The listing builds one solid part. Answer for the finished solid, in the listing's coordinates (mm). Face numbers are marked on the shaded views. Round coordinates to 2 decimals unless told otherwise and drop trailing zeros. Order: outer loops, then holes, each group sorted by start corner. A loop starts at its lowest first (then second) coordinate and runs counter-clockwise, first axis right, second up. Notation, with made-up numbers: (75, 87) -> (125, 87) arc R21 cw to (125, 103) -> close; hole circle Ø11 at (-21, 86). An arc over 180 degrees is marked (long way). Answer in a Markdown table with one row per item. Add a question column.
```python
from build123d import *
from build123d.topology import SkipClean

# Parameters (mm, degrees)
SKETCH1_R           = 76.2
BOSS_EXTRUDE1_DEPTH = 6.35
CUT_EXTRUDE2_START  = -6.35
SKETCH2_R           = 4.7625
SKETCH2_R_2         = 19.05
CUT_EXTRUDE2_DEPTH  = 6.35
BOSS_EXTRUDE2_DEPTH = 3
SKETCH4_R           = 1.5
SKETCH4_R_2         = 1.25
CUT_EXTRUDE3_DEPTH  = 86.348763
FILLET1_R           = 2.54
SKETCH5_R           = 2.5
CUT_EXTRUDE4_DEPTH  = 2.85


with BuildPart() as part:
    # Sketch1 → Boss-Extrude1 (new body)
    with BuildSketch(Plane(origin=(0, 0, 0), x_dir=(1, 0, 0), z_dir=(0, 1, 0))):
        with Locations(Location((0, 0, 0), (0, 0, 270))):
            Circle(SKETCH1_R)
    extrude(amount=BOSS_EXTRUDE1_DEPTH)

    # Sketch2 → Cut-Extrude2 (cut)
    with BuildSketch(Plane(origin=(0, 6.35, 0), x_dir=(1, 0, 0), z_dir=(0, 1, 0)).offset(CUT_EXTRUDE2_START)):
        with BuildLine():
            ThreePointArc((61.150771, -23.195291), (0, -37.290064), (-61.150771, -23.195291))
            ThreePointArc((-61.150771, -23.195291), (-72.108092, -13.824804), (-76.2, 0))
            ThreePointArc((-76.2, 0), (0, -76.2), (76.2, 0))
            ThreePointArc((76.2, 0), (72.108092, -13.824804), (61.150771, -23.195291))
        make_face()
        with BuildLine():
            ThreePointArc((-61.150771, 23.195291), (0, 37.290064), (61.150771, 23.195291))
            ThreePointArc((61.150771, 23.195291), (72.108092, 13.824804), (76.2, 0))
            ThreePointArc((76.2, 0), (0, 76.2), (-76.2, 0))
            ThreePointArc((-76.2, 0), (-72.108092, 13.824804), (-61.150771, 23.195291))
        make_face()
        with Locations(Location((-50.8, 0, 0), (0, 0, 270))):
            Circle(SKETCH2_R)
        with Locations(Location((50.8, 0, 0), (0, 0, 270))):
            Circle(SKETCH2_R)
        with Locations(Location((0, 0, 0), (0, 0, 270))):
            Circle(SKETCH2_R_2)
    extrude(amount=CUT_EXTRUDE2_DEPTH, mode=Mode.SUBTRACT)

    # Sketch3 → Boss-Extrude2 (add)
    with SkipClean():  # the faces are left unmerged after this step: merging them gives an invalid solid
        with BuildSketch(Plane(origin=(0, 6.35, 0), x_dir=(1, 0, 0), z_dir=(0, 1, 0))):
            with BuildLine():
                Line((-38.5, 4.75), (-38.5, -4.75))
                Line((-38.5, -4.75), (-38.5, -11.25))
                Line((-38.5, -11.25), (-38.5, -16))
                Line((-38.5, -16), (-18, -16))
                Line((-18, -16), (-11.5, -16))
                Line((-11.5, -16), (-10.339367, -16))
                ThreePointArc((-10.339367, -16), (-13.611535, -13.327739), (-16.214268, -10))
                Line((-16.214268, -10), (-31.096327, -10))
                Line((-31.096327, -10), (-32.5, -10))
                Line((-32.5, -10), (-32.5, -8.522949))
                Line((-32.5, -8.522949), (-32.5, 8.425596))
                Line((-32.5, 8.425596), (-32.5, 10))
                Line((-32.5, 10), (-31.027855, 10))
                Line((-31.027855, 10), (-16.214268, 10))
                ThreePointArc((-16.214268, 10), (-13.611535, 13.327739), (-10.339367, 16))
                Line((-10.339367, 16), (-11.5, 16))
                Line((-11.5, 16), (-18, 16))
                Line((-18, 16), (-38.5, 16))
                Line((-38.5, 16), (-38.5, 11.25))
                Line((-38.5, 11.25), (-38.5, 4.75))
            make_face()
        extrude(amount=BOSS_EXTRUDE2_DEPTH)

    # Sketch4 → Cut-Extrude3 (cut, through all)
    # profile 1 of 12: a face of its own
    with SkipClean():  # the faces are left unmerged after this step: merging them gives an invalid solid
        with BuildSketch(Plane(origin=(0, 9.35, 0), x_dir=(1, 0, 0), z_dir=(0, 1, 0))):
            with Locations(Location((-30.75, -13.5, 0), (0, 0, 270))):
                Circle(SKETCH4_R)
            with Locations((-30.75, -13.5)):
                Circle(SKETCH4_R_2, mode=Mode.SUBTRACT)
        # profile 2 of 12: a face of its own
        with BuildSketch(Plane(origin=(0, 9.35, 0), x_dir=(1, 0, 0), z_dir=(0, 1, 0))):
            with Locations((-30.75, -13.5)):
                Circle(SKETCH4_R_2)
        # profile 3 of 12: a face of its own
        with BuildSketch(Plane(origin=(0, 9.35, 0), x_dir=(1, 0, 0), z_dir=(0, 1, 0))):
            with Locations(Location((-22.75, -13.5, 0), (0, 0, 270))):
                Circle(SKETCH4_R)
            with Locations((-22.75, -13.5)):
                Circle(SKETCH4_R_2, mode=Mode.SUBTRACT)
        # profile 4 of 12: a face of its own
        with BuildSketch(Plane(origin=(0, 9.35, 0), x_dir=(1, 0, 0), z_dir=(0, 1, 0))):
            with Locations((-22.75, -13.5)):
                Circle(SKETCH4_R_2)
        # profile 5 of 12: a face of its own
        with BuildSketch(Plane(origin=(0, 9.35, 0), x_dir=(1, 0, 0), z_dir=(0, 1, 0))):
            with Locations(Location((-36, -8, 0), (0, 0, 270))):
                Circle(SKETCH4_R)
            with Locations((-36, -8)):
                Circle(SKETCH4_R_2, mode=Mode.SUBTRACT)
        # profile 6 of 12: a face of its own
        with BuildSketch(Plane(origin=(0, 9.35, 0), x_dir=(1, 0, 0), z_dir=(0, 1, 0))):
            with Locations((-36, -8)):
                Circle(SKETCH4_R_2)
        # profile 7 of 12: a face of its own
        with BuildSketch(Plane(origin=(0, 9.35, 0), x_dir=(1, 0, 0), z_dir=(0, 1, 0))):
            with Locations(Location((-36, 8, 0), (0, 0, 270))):
                Circle(SKETCH4_R)
            with Locations((-36, 8)):
                Circle(SKETCH4_R_2, mode=Mode.SUBTRACT)
        # profile 8 of 12: a face of its own
        with BuildSketch(Plane(origin=(0, 9.35, 0), x_dir=(1, 0, 0), z_dir=(0, 1, 0))):
            with Locations((-36, 8)):
                Circle(SKETCH4_R_2)
        # profile 9 of 12: a face of its own
        with BuildSketch(Plane(origin=(0, 9.35, 0), x_dir=(1, 0, 0), z_dir=(0, 1, 0))):
            with Locations(Location((-30.75, 13.5, 0), (0, 0, 270))):
                Circle(SKETCH4_R)
            with Locations((-30.75, 13.5)):
                Circle(SKETCH4_R_2, mode=Mode.SUBTRACT)
        # profile 10 of 12: a face of its own
        with BuildSketch(Plane(origin=(0, 9.35, 0), x_dir=(1, 0, 0), z_dir=(0, 1, 0))):
            with Locations((-30.75, 13.5)):
                Circle(SKETCH4_R_2)
        # profile 11 of 12: a face of its own
        with BuildSketch(Plane(origin=(0, 9.35, 0), x_dir=(1, 0, 0), z_dir=(0, 1, 0))):
            with Locations(Location((-22.75, 13.5, 0), (0, 0, 270))):
                Circle(SKETCH4_R)
            with Locations((-22.75, 13.5)):
                Circle(SKETCH4_R_2, mode=Mode.SUBTRACT)
        # profile 12 of 12: a face of its own
        with BuildSketch(Plane(origin=(0, 9.35, 0), x_dir=(1, 0, 0), z_dir=(0, 1, 0))):
            with Locations((-22.75, 13.5)):
                Circle(SKETCH4_R_2)
        extrude(amount=-CUT_EXTRUDE3_DEPTH, mode=Mode.SUBTRACT)

    # Fillet1
    # the kernel refuses this fillet: 2.54 mm, written as the material it adds along each edge
    with BuildSketch(Plane(origin=(-3.989367, 6.35, -16), x_dir=(0, 0, -1), z_dir=(-1, 0, 0))) as fillet1_piece_1_section:
        with BuildLine():
            CenterArc((FILLET1_R, -FILLET1_R), FILLET1_R, 90, 90)
            Line((0, -FILLET1_R), (0, 0))
            Line((0, 0), (FILLET1_R, 0))
        make_face()
    fillet1_piece_1 = extrude(amount=34.510633, mode=Mode.PRIVATE)
    fillet1_piece_1 = fillet1_piece_1 - Plane(origin=(0, 6.913548, 0), x_dir=(0, 0, 1), z_dir=(0, -1, 0)) * Cylinder(19.05, 80, mode=Mode.PRIVATE)
    add(fillet1_piece_1)
    with BuildSketch(Plane(origin=(-38.5, 6.35, 16), x_dir=(0, 0, 1), z_dir=(1, 0, 0))) as fillet1_piece_2_section:
        with BuildLine():
            CenterArc((FILLET1_R, -FILLET1_R), FILLET1_R, 90, 90)
            Line((0, -FILLET1_R), (0, 0))
            Line((0, 0), (FILLET1_R, 0))
        make_face()
    fillet1_piece_2 = extrude(amount=34.510633, mode=Mode.PRIVATE)
    fillet1_piece_2 = fillet1_piece_2 - Plane(origin=(0, 6.913549, 0), x_dir=(0, 0, 1), z_dir=(0, -1, 0)) * Cylinder(19.05, 80, mode=Mode.PRIVATE)
    add(fillet1_piece_2)
    with BuildSketch(Plane(origin=(-38.5, 6.35, -16), x_dir=(-1, 0, 0), z_dir=(0, 0, 1))) as fillet1_piece_3:
        with BuildLine():
            CenterArc((FILLET1_R, -FILLET1_R), FILLET1_R, 90, 90)
            Line((0, -FILLET1_R), (0, 0))
            Line((0, 0), (FILLET1_R, 0))
        make_face()
    extrude(amount=32)
    with BuildSketch(Plane(origin=(-3.989367, 6.35, -16), x_dir=(0, 0, -1), z_dir=(-1, 0, 0))) as fillet1_piece_4a_section:
        with BuildLine():
            CenterArc((FILLET1_R, -FILLET1_R), FILLET1_R, 90, 90)
            Line((0, -FILLET1_R), (0, 0))
            Line((0, 0), (FILLET1_R, 0))
        make_face()
    fillet1_piece_4a = extrude(amount=40.860633, mode=Mode.PRIVATE)
    fillet1_piece_4a = split(fillet1_piece_4a, bisect_by=Plane(origin=(-38.5, 6.925044, -16.575044), z_dir=(-1, 0, 0)), keep=Keep.TOP, mode=Mode.PRIVATE)
    with BuildSketch(Plane(origin=(-38.5, 6.35, -22.35), x_dir=(-1, 0, 0), z_dir=(0, 0, 1))) as fillet1_piece_4b_section:
        with BuildLine():
            CenterArc((FILLET1_R, -FILLET1_R), FILLET1_R, 90, 90)
            Line((0, -FILLET1_R), (0, 0))
            Line((0, 0), (FILLET1_R, 0))
        make_face()
    fillet1_piece_4b = extrude(amount=38.35, mode=Mode.PRIVATE)
    fillet1_piece_4b = split(fillet1_piece_4b, bisect_by=Plane(origin=(-39.075044, 6.925044, -16), z_dir=(0, 0, -1)), keep=Keep.TOP, mode=Mode.PRIVATE)
    fillet1_piece_4 = fillet1_piece_4a & fillet1_piece_4b
    add(fillet1_piece_4)
    with BuildSketch(Plane(origin=(-38.5, 6.35, -16), x_dir=(-1, 0, 0), z_dir=(0, 0, 1))) as fillet1_piece_5a_section:
        with BuildLine():
            CenterArc((FILLET1_R, -FILLET1_R), FILLET1_R, 90, 90)
            Line((0, -FILLET1_R), (0, 0))
            Line((0, 0), (FILLET1_R, 0))
        make_face()
    fillet1_piece_5a = extrude(amount=38.35, mode=Mode.PRIVATE)
    fillet1_piece_5a = split(fillet1_piece_5a, bisect_by=Plane(origin=(-39.075044, 6.925044, 16), z_dir=(0, 0, 1)), keep=Keep.TOP, mode=Mode.PRIVATE)
    with BuildSketch(Plane(origin=(-44.85, 6.35, 16), x_dir=(0, 0, 1), z_dir=(1, 0, 0))) as fillet1_piece_5b_section:
        with BuildLine():
            CenterArc((FILLET1_R, -FILLET1_R), FILLET1_R, 90, 90)
            Line((0, -FILLET1_R), (0, 0))
            Line((0, 0), (FILLET1_R, 0))
        make_face()
    fillet1_piece_5b = extrude(amount=40.860633, mode=Mode.PRIVATE)
    fillet1_piece_5b = split(fillet1_piece_5b, bisect_by=Plane(origin=(-38.5, 6.925044, 16.575044), z_dir=(-1, 0, 0)), keep=Keep.TOP, mode=Mode.PRIVATE)
    fillet1_piece_5 = fillet1_piece_5a & fillet1_piece_5b
    add(fillet1_piece_5)

    # Sketch5 → Cut-Extrude4 (cut)
    with BuildSketch(Plane.XZ):
        with Locations(Location((-22.75, 13.5, 0), (0, 0, 270))):
            Circle(SKETCH5_R)
        with Locations(Location((-30.75, 13.5, 0), (0, 0, 270))):
            Circle(SKETCH5_R)
        with Locations(Location((-36, 8, 0), (0, 0, 270))):
            Circle(SKETCH5_R)
        with Locations(Location((-36, -8, 0), (0, 0, 270))):
            Circle(SKETCH5_R)
        with Locations(Location((-30.75, -13.5, 0), (0, 0, 270))):
            Circle(SKETCH5_R)
        with Locations(Location((-22.75, -13.5, 0), (0, 0, 270))):
            Circle(SKETCH5_R)
    extrude(amount=-CUT_EXTRUDE4_DEPTH, mode=Mode.SUBTRACT)


solid = part.part
```
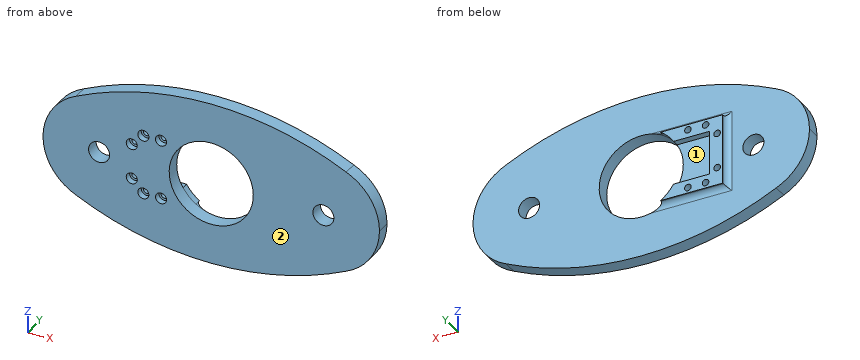
1. The part is cut by section B-B (y = 4.5). Give the number of separate pieces and of enclosed holes in the cut face, then the cut area to 3 significant figures.
2. Each of these flat-tipped pins is pushed along its axis until it touches: pin 1 (6.5 mm diameter, centred on x = -36, z = -8, fed in from +Y); pin 2 (3 mm diameter, centred on y = 2, z = -17, fed in from -X); pin 3 (0.9 mm diameter, centred on y = 7.5, z = 0.5, fed in from +X); pin 4 (2 mm diameter, centred on x = -54.5, y = 2.5, fed in from -Z). Where does it stop, or does it pass through?
3. The part is cut by section C-C (z = 1.5). Give the vertices of the cut face in (x, y).
4. The part is cut by section A-A (x = 0). Give the vertices of the cut face in (y, z).
5. Straight lines are drawn through the part: line 1 along X through (y, z) = (0.75, -3); line 2 along X through (y, z) = (1.5, -14); line 3 along Y through (x, z) = (22.5, 24.5). For each, find the intervals that lie inside material, in ascending order.
6. The mould has two halves that part along Z. Classify the marked faces 1 and 2: released by +Z, released by -Z, zero draft, split by the parting line, or undercut.
Report:
| question | item | result |
|---|---|---|
| 1 | separate pieces | 1 |
| 1 | enclosed holes | 9 |
| 1 | area | 7,680 mm^2 |
| 2 | pin 1 | stops at y = 9.35 |
| 2 | pin 2 | stops at x = -70.92 |
| 2 | pin 3 | stops at x = -32.5 |
| 2 | pin 4 | stops at z = -26.64 |
| 3 | outline | (-76.16, 0) -> (-55.32, 0) -> (-55.32, 6.35) -> (-76.16, 6.35) -> close; (-46.28, 0) -> (-18.99, 0) -> (-18.99, 6.35) -> (-32.5, 6.35) -> (-32.5, 9.35) -> (-38.5, 9.35) -> (-38.5, 8.89) arc R2.54 cw to (-41.04, 6.35) -> (-46.28, 6.35) -> close; (18.99, 0) -> (46.28, 0) -> (46.28, 6.35) -> (18.99, 6.35) -> close; (55.32, 0) -> (76.16, 0) -> (76.16, 6.35) -> (55.32, 6.35) -> close |
| 4 | outline | (0, -37.29) -> (6.35, -37.29) -> (6.35, -19.05) -> (0, -19.05) -> close; (0, 19.05) -> (6.35, 19.05) -> (6.35, 37.29) -> (0, 37.29) -> close |
| 5 | line 1 | x = -76.02 to -54.5, -47.1 to -18.81, 18.81 to 47.1, 54.5 to 76.02 |
| 5 | line 2 | x = -71.99 to -33.2, -28.3 to -25.2, -20.3 to -12.92, 12.92 to 71.99 |
| 5 | line 3 | y = 0 to 6.35 |
| 6 | face 1 | undercut |
| 6 | face 2 | zero draft |
